The listing builds one solid part. Answer for the finished solid, in the listing's coordinates (mm). A direction names the side the tool comes from. Give positions to 0.01 mm unless a question says otherwise; leave off trailing zeros. Write each loop counter-clockwise with the first axis right and the second up, starting at its lowest first coordinate (ties: lowest second). Pieces come first, ordered by that corner, then holes.
```python
from build123d import *

# Parameters (mm, degrees)
SKETCH_W     = 25
SKETCH_H     = 25
SKETCH_W_2   = 22
SKETCH_H_2   = 22
PAD_DEPTH    = 584
FILLET_R     = 0.74
POCKET_DEPTH = 25.001


with BuildPart() as part:
    # Sketch → Pad (new body)
    with BuildSketch(Plane.XY):
        with Locations((12.5, 12.5)):
            Rectangle(SKETCH_W, SKETCH_H)
        with Locations((12.5, 12.5)):
            Rectangle(SKETCH_W_2, SKETCH_H_2, mode=Mode.SUBTRACT)
    extrude(amount=PAD_DEPTH)

    # Fillet
    fillet_edges = [part.edges().sort_by_distance(p)[0] for p in [
        (25, 0, 292),
        (0, 0, 292),
        (25, 25, 292),
        (0, 25, 292),
    ]]
    fillet(fillet_edges, radius=FILLET_R)

    # Sketch001 (on Face6 of Fillet) → Pocket (cut, through all)
    with BuildSketch(Plane(origin=(0, 0, 0), x_dir=(0, -1, 0), z_dir=(-1, 0, 0))):
        Polygon((0, 0), (-42.305785, 7.459651), (-25.0585, -14.483582), align=None)
        Polygon((-25, 584), (31.802426, 573.9842), (24.213916, 600.392365), align=None)
    extrude(amount=-POCKET_DEPTH, mode=Mode.SUBTRACT)


solid = part.part
```
Item 1: A cutting plane is placed at A-A, the plane x = 11.5. Give the vertices of the cut face in (y, z).
Conclusion:
outline: (0, 0) - (1.5, 0.26) - (1.5, 579.86) - (0, 579.59) - close; (23.5, 4.14) - (25, 4.41) - (25, 584) - (23.5, 583.74) - close
Item 2: A cutting plane is placed at B-B, the plane z = 198.5. Give the vertices of the cut face in (x, y), plus the area to 3 significant figures.
Conclusion:
outline: (0, 0.74) arc R0.74 ccw to (0.74, 0) - (24.26, 0) arc R0.74 ccw to (25, 0.74) - (25, 24.26) arc R0.74 ccw to (24.26, 25) - (0.74, 25) arc R0.74 ccw to (0, 24.26) - close; hole (1.5, 1.5) - (23.5, 1.5) - (23.5, 23.5) - (1.5, 23.5) - close
area: 141 mm2
Item 3: A cutting plane is placed at C-C, the plane y = 11.25. Give the vertices of the cut face in (x, z), plus the area to 3 significant figures.
Conclusion:
outline: (0, 1.98) - (1.5, 1.98) - (1.5, 581.58) - (0, 581.58) - close; (23.5, 1.98) - (25, 1.98) - (25, 581.58) - (23.5, 581.58) - close
area: 1,740 mm2
Item 4: Determine the mould class of faces 3 (the face through (12, 0, 286)), 4 (the face through (25, 12, 288)), 5 (the face through (23.5, 12, 288)) for opening direction Y: pulls with the +Y half, pulls with the -Y half, needs draft (parallel to the pull), parting line crosses it, or undercut.
Conclusion:
face 3: pulls with the -Y half
face 4: needs draft
face 5: undercut
Item 5: Each of these flat-tipped pins is pushed along its axis until it touches: P1, Ø10, axis at x = 4, y = 11, coming from the +Z side; P2, Ø12, axis at x = 21.5, y = 22, coming from the -Z side. Where does it stop, or does it pass through?
Conclusion:
P1: stops at z = 582.29
P2: stops at z = 2.88
Item 6: Consider probe 1 along X at (y, z) = (14.25, 213.5); probe 2 along Z at (x, y) = (12.75, 24). Determine where each line is inside the solid, lowest interval first.
Conclusion:
probe 1: x = 0 to 1.5, 23.5 to 25
probe 2: z = 4.23 to 583.82
Item 7: Which of the six approach directions +Z, -Z, +X, -X, +Y, -Y give full straight-line access (tool end or side, diameter ignored) to faces 1 (the face through (12, 23.5, 290)), 2 (the face through (1.331, 12.442, 2.194))?
Conclusion:
face 1: +Z, -Z
face 2: -Z, +X, -X, +Y
